Could you check a few things on this model? Use its own coordinates, in mm. Give positions to 0.01 mm unless a question says otherwise; leave off trailing zeros. Loops run counter-clockwise (first coordinate to the right, second up) from the corner with the lowest first, then second, coordinate; pieces in that order, holes last.
1. I need wall thicknesses on line 1 along Z through (x, y) = (10, -8.9); line 2 along Y through (x, z) = (-8, 18); line 3 along X through (y, z) = (-8.9, 160). Which ranges of each line are inside material? Lowest first, please.
2. Imagine slicing it at D-D (z = 180). Count the separate pieces of the cut face and the enclosed holes in it, plus the area to 3 significant figures.
3. Imagine slicing it at C-C (x = 10). List the corners of the cut face in (y, z) for me, plus the area to 3 significant figures.
4. Imagine slicing it at B-B (x = 0). List the corners of the cut face in (y, z) for me, plus the area to 3 significant figures.
5. For P1, Ø3, axis at y = 1, z = 99, coming from the -X side; P2, Ø0.6, axis at y = 9, z = 52.5, coming from the +X side, each with a flat end and sliding along its axis, tell me the tip position at first contact or that it passes through.
6. Imagine slicing it at A-A (y = 0). List the corners of the cut face in (x, z) for me.
```python
from build123d import *

# Parameters (mm, degrees)
BOSS_EXTRUDE1_DEPTH = 200
SKETCH2_R           = 2.5
CUT_EXTRUDE1_DEPTH  = 203.484567313
SKETCH3_R           = 2
CUT_EXTRUDE2_DEPTH  = 40


with BuildPart() as part:
    # Sketch1 → Boss-Extrude1 (new body)
    with BuildSketch(Plane.XY):
        with BuildLine():
            Line((-8.5, 10), (-3.8, 10))
            ThreePointArc((-3.8, 10), (-3.658578644, 9.941421356), (-3.6, 9.8))
            Line((-3.6, 9.8), (-3.6, 9.7))
            ThreePointArc((-3.6, 9.7), (-3.541421356, 9.558578644), (-3.4, 9.5))
            Line((-3.4, 9.5), (-3.3, 9.5))
            ThreePointArc((-3.3, 9.5), (-3.158578644, 9.441421356), (-3.1, 9.3))
            Line((-3.1, 9.3), (3.1, 9.3))
            ThreePointArc((3.1, 9.3), (3.158578644, 9.441421356), (3.3, 9.5))
            Line((3.3, 9.5), (3.4, 9.5))
            ThreePointArc((3.4, 9.5), (3.541421356, 9.558578644), (3.6, 9.7))
            Line((3.6, 9.7), (3.6, 9.8))
            ThreePointArc((3.6, 9.8), (3.658578644, 9.941421356), (3.8, 10))
            Line((3.8, 10), (8.5, 10))
            Line((8.5, 10), (11.5, 10))
            Line((11.5, 10), (16.2, 10))
            ThreePointArc((16.2, 10), (16.341421356, 9.941421356), (16.4, 9.8))
            Line((16.4, 9.8), (16.4, 9.7))
            ThreePointArc((16.4, 9.7), (16.458578644, 9.558578644), (16.6, 9.5))
            Line((16.6, 9.5), (16.7, 9.5))
            ThreePointArc((16.7, 9.5), (16.841421356, 9.441421356), (16.9, 9.3))
            Line((16.9, 9.3), (16.9, 8.2))
            Line((16.9, 8.2), (14.7, 8.2))
            ThreePointArc((14.7, 8.2), (14.558578644, 8.141421356), (14.5, 8))
            Line((14.5, 8), (14.5, 6.560660172))
            Line((14.5, 6.560660172), (17.102081528, 3.958578644))
            ThreePointArc((17.102081528, 3.958578644), (17.166966198, 3.915224093), (17.243502884, 3.9))
            Line((17.243502884, 3.9), (22.756497116, 3.9))
            ThreePointArc((22.756497116, 3.9), (22.833033802, 3.915224093), (22.897918472, 3.958578644))
            Line((22.897918472, 3.958578644), (25.5, 6.560660172))
            Line((25.5, 6.560660172), (25.5, 8))
            ThreePointArc((25.5, 8), (25.441421356, 8.141421356), (25.3, 8.2))
            Line((25.3, 8.2), (23.1, 8.2))
            Line((23.1, 8.2), (23.1, 9.3))
            ThreePointArc((23.1, 9.3), (23.158578644, 9.441421356), (23.3, 9.5))
            Line((23.3, 9.5), (23.4, 9.5))
            ThreePointArc((23.4, 9.5), (23.541421356, 9.558578644), (23.6, 9.7))
            Line((23.6, 9.7), (23.6, 9.8))
            ThreePointArc((23.6, 9.8), (23.658578644, 9.941421356), (23.8, 10))
            Line((23.8, 10), (28.5, 10))
            ThreePointArc((28.5, 10), (29.560660172, 9.560660172), (30, 8.5))
            Line((30, 8.5), (30, 3.8))
            ThreePointArc((30, 3.8), (29.941421356, 3.658578644), (29.8, 3.6))
            Line((29.8, 3.6), (29.7, 3.6))
            ThreePointArc((29.7, 3.6), (29.558578644, 3.541421356), (29.5, 3.4))
            Line((29.5, 3.4), (29.5, 3.3))
            ThreePointArc((29.5, 3.3), (29.441421356, 3.158578644), (29.3, 3.1))
            Line((29.3, 3.1), (28.2, 3.1))
            Line((28.2, 3.1), (28.2, 5.3))
            ThreePointArc((28.2, 5.3), (28.141421356, 5.441421356), (28, 5.5))
            Line((28, 5.5), (26.560660172, 5.5))
            Line((26.560660172, 5.5), (23.958578644, 2.897918472))
            ThreePointArc((23.958578644, 2.897918472), (23.915224093, 2.833033802), (23.9, 2.756497116))
            Line((23.9, 2.756497116), (23.9, -2.756497116))
            ThreePointArc((23.9, -2.756497116), (23.915224093, -2.833033802), (23.958578644, -2.897918472))
            Line((23.958578644, -2.897918472), (26.560660172, -5.5))
            Line((26.560660172, -5.5), (28, -5.5))
            ThreePointArc((28, -5.5), (28.141421356, -5.441421356), (28.2, -5.3))
            Line((28.2, -5.3), (28.2, -3.1))
            Line((28.2, -3.1), (29.3, -3.1))
            ThreePointArc((29.3, -3.1), (29.441421356, -3.158578644), (29.5, -3.3))
            Line((29.5, -3.3), (29.5, -3.4))
            ThreePointArc((29.5, -3.4), (29.558578644, -3.541421356), (29.7, -3.6))
            Line((29.7, -3.6), (29.8, -3.6))
            ThreePointArc((29.8, -3.6), (29.941421356, -3.658578644), (30, -3.8))
            Line((30, -3.8), (30, -8.5))
            ThreePointArc((30, -8.5), (29.560660172, -9.560660172), (28.5, -10))
            Line((28.5, -10), (23.8, -10))
            ThreePointArc((23.8, -10), (23.658578644, -9.941421356), (23.6, -9.8))
            Line((23.6, -9.8), (23.6, -9.7))
            ThreePointArc((23.6, -9.7), (23.541421356, -9.558578644), (23.4, -9.5))
            Line((23.4, -9.5), (23.3, -9.5))
            ThreePointArc((23.3, -9.5), (23.158578644, -9.441421356), (23.1, -9.3))
            Line((23.1, -9.3), (23.1, -8.2))
            Line((23.1, -8.2), (25.3, -8.2))
            ThreePointArc((25.3, -8.2), (25.441421356, -8.141421356), (25.5, -8))
            Line((25.5, -8), (25.5, -6.560660172))
            Line((25.5, -6.560660172), (22.897918472, -3.958578644))
            ThreePointArc((22.897918472, -3.958578644), (22.833033802, -3.915224093), (22.756497116, -3.9))
            Line((22.756497116, -3.9), (17.243502884, -3.9))
            ThreePointArc((17.243502884, -3.9), (17.166966198, -3.915224093), (17.102081528, -3.958578644))
            Line((17.102081528, -3.958578644), (14.5, -6.560660172))
            Line((14.5, -6.560660172), (14.5, -8))
            ThreePointArc((14.5, -8), (14.558578644, -8.141421356), (14.7, -8.2))
            Line((14.7, -8.2), (16.9, -8.2))
            Line((16.9, -8.2), (16.9, -9.3))
            ThreePointArc((16.9, -9.3), (16.841421356, -9.441421356), (16.7, -9.5))
            Line((16.7, -9.5), (16.6, -9.5))
            ThreePointArc((16.6, -9.5), (16.458578644, -9.558578644), (16.4, -9.7))
            Line((16.4, -9.7), (16.4, -9.8))
            ThreePointArc((16.4, -9.8), (16.341421356, -9.941421356), (16.2, -10))
            Line((16.2, -10), (11.5, -10))
            Line((11.5, -10), (8.5, -10))
            Line((8.5, -10), (3.8, -10))
            ThreePointArc((3.8, -10), (3.658578644, -9.941421356), (3.6, -9.8))
            Line((3.6, -9.8), (3.6, -9.7))
            ThreePointArc((3.6, -9.7), (3.541421356, -9.558578644), (3.4, -9.5))
            Line((3.4, -9.5), (3.3, -9.5))
            Line((3.3, -9.5), (-3.3, -9.5))
            Line((-3.3, -9.5), (-3.4, -9.5))
            ThreePointArc((-3.4, -9.5), (-3.541421356, -9.558578644), (-3.6, -9.7))
            Line((-3.6, -9.7), (-3.6, -9.8))
            ThreePointArc((-3.6, -9.8), (-3.658578644, -9.941421356), (-3.8, -10))
            Line((-3.8, -10), (-8.5, -10))
            ThreePointArc((-8.5, -10), (-9.560660172, -9.560660172), (-10, -8.5))
            Line((-10, -8.5), (-10, -3.8))
            ThreePointArc((-10, -3.8), (-9.941421356, -3.658578644), (-9.8, -3.6))
            Line((-9.8, -3.6), (-9.7, -3.6))
            ThreePointArc((-9.7, -3.6), (-9.558578644, -3.541421356), (-9.5, -3.4))
            Line((-9.5, -3.4), (-9.5, -3.3))
            ThreePointArc((-9.5, -3.3), (-9.441421356, -3.158578644), (-9.3, -3.1))
            Line((-9.3, -3.1), (-8.2, -3.1))
            Line((-8.2, -3.1), (-8.2, -5.3))
            ThreePointArc((-8.2, -5.3), (-8.141421356, -5.441421356), (-8, -5.5))
            Line((-8, -5.5), (-6.560660172, -5.5))
            Line((-6.560660172, -5.5), (-3.958578644, -2.897918472))
            ThreePointArc((-3.958578644, -2.897918472), (-3.915224093, -2.833033802), (-3.9, -2.756497116))
            Line((-3.9, -2.756497116), (-3.9, 2.756497116))
            ThreePointArc((-3.9, 2.756497116), (-3.915224093, 2.833033802), (-3.958578644, 2.897918472))
            Line((-3.958578644, 2.897918472), (-6.560660172, 5.5))
            Line((-6.560660172, 5.5), (-8, 5.5))
            ThreePointArc((-8, 5.5), (-8.141421356, 5.441421356), (-8.2, 5.3))
            Line((-8.2, 5.3), (-8.2, 3.1))
            Line((-8.2, 3.1), (-9.3, 3.1))
            ThreePointArc((-9.3, 3.1), (-9.441421356, 3.158578644), (-9.5, 3.3))
            Line((-9.5, 3.3), (-9.5, 3.4))
            ThreePointArc((-9.5, 3.4), (-9.558578644, 3.541421356), (-9.7, 3.6))
            Line((-9.7, 3.6), (-9.8, 3.6))
            ThreePointArc((-9.8, 3.6), (-9.941421356, 3.658578644), (-10, 3.8))
            Line((-10, 3.8), (-10, 8.5))
            ThreePointArc((-10, 8.5), (-9.560660172, 9.560660172), (-8.5, 10))
        make_face()
        with BuildLine():
            Line((3.9, 2.756497116), (3.9, -2.756497116))
            ThreePointArc((3.9, -2.756497116), (3.915224093, -2.833033802), (3.958578644, -2.897918472))
            Line((3.958578644, -2.897918472), (6.560660172, -5.5))
            Line((6.560660172, -5.5), (6.560660172, -8.2))
            Line((6.560660172, -8.2), (13.439339828, -8.2))
            Line((13.439339828, -8.2), (13.439339828, -5.5))
            Line((13.439339828, -5.5), (16.041421356, -2.897918472))
            ThreePointArc((16.041421356, -2.897918472), (16.084775907, -2.833033802), (16.1, -2.756497116))
            Line((16.1, -2.756497116), (16.1, 2.756497116))
            ThreePointArc((16.1, 2.756497116), (16.084775907, 2.833033802), (16.041421356, 2.897918472))
            Line((16.041421356, 2.897918472), (13.439339828, 5.5))
            Line((13.439339828, 5.5), (13.439339828, 8.2))
            Line((13.439339828, 8.2), (6.560660172, 8.2))
            Line((6.560660172, 8.2), (6.560660172, 5.5))
            Line((6.560660172, 5.5), (3.958578644, 2.897918472))
            ThreePointArc((3.958578644, 2.897918472), (3.915224093, 2.833033802), (3.9, 2.756497116))
        make_face(mode=Mode.SUBTRACT)
    extrude(amount=BOSS_EXTRUDE1_DEPTH)

    # Sketch2 → Cut-Extrude1 (cut, through all)
    with BuildSketch(Plane.XY.offset(200)):
        Circle(SKETCH2_R)
        with Locations(Location((20, 0, 0), (0, 0, 180))):
            Circle(SKETCH2_R)
    extrude(amount=-CUT_EXTRUDE1_DEPTH, mode=Mode.SUBTRACT)

    # Sketch3 → Cut-Extrude2 (cut)
    with BuildSketch(Plane(origin=(0, -10, 0), x_dir=(-1, 0, 0), z_dir=(0, -1, 0))):
        with Locations(Location((-10, -180, 0), (0, 0, 180))):
            Circle(SKETCH3_R)
        with Locations(Location((-10, -160, 0), (0, 0, 180))):
            Circle(SKETCH3_R)
    extrude(amount=-CUT_EXTRUDE2_DEPTH, mode=Mode.SUBTRACT)


solid = part.part
```
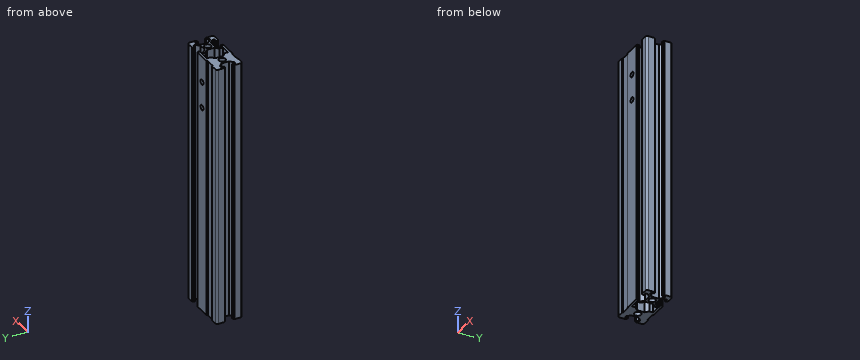
Derived:
1. line 1: z = 0 to 158, 162 to 178, 182 to 200
1. line 2: y = -10 to -5.5, 5.5 to 10
1. line 3: x = -9.95 to 8, 12 to 16.9, 23.1 to 29.95
2. separate pieces: 2
2. enclosed holes: 2
2. area: 371 mm2
3. outline: (-10, 0) - (-8.2, 0) - (-8.2, 158) - (-10, 158) - close; (-10, 162) - (-8.2, 162) - (-8.2, 178) - (-10, 178) - close; (-10, 182) - (-8.2, 182) - (-8.2, 200) - (-10, 200) - close; (8.2, 0) - (10, 0) - (10, 158) - (8.2, 158) - close; (8.2, 162) - (10, 162) - (10, 178) - (8.2, 178) - close; (8.2, 182) - (10, 182) - (10, 200) - (8.2, 200) - close
3. area: 691 mm2
4. outline: (-9.5, 0) - (-2.5, 0) - (-2.5, 200) - (-9.5, 200) - close; (2.5, 0) - (9.3, 0) - (9.3, 200) - (2.5, 200) - close
4. area: 2,760 mm2
5. P1: stops at x = -3.9
5. P2: stops at x = 29.99
6. outline: (-3.9, 0) - (-2.5, 0) - (-2.5, 200) - (-3.9, 200) - close; (2.5, 0) - (3.9, 0) - (3.9, 200) - (2.5, 200) - close; (16.1, 0) - (17.5, 0) - (17.5, 200) - (16.1, 200) - close; (22.5, 0) - (23.9, 0) - (23.9, 200) - (22.5, 200) - close
